from build123d import *

# Parameters (mm, degrees)
F3_DEPTH = 3.15
F4_R     = 0.79999
F5_R     = 0.6


# Not quite as in the source:
# - a fillet or chamfer is up to 0.001 mm smaller than in the source, because OpenCascade refuses the exact size


with BuildPart() as f1:
    # F0 (on Front) → F1 (revolve)
    with BuildSketch(Plane.XZ):
        Polygon((0, 24.5), (0, 0), (4, 0), (4, 15), (2.5, 15), (2.5, 24.5), align=None)
    revolve(axis=Axis((0, 0, -0.3548332296), (0, 0, -1)))

    # F2 (on Front) → F3 (join, symmetric)
    with BuildSketch(Plane.XZ):
        with BuildLine():
            ThreePointArc((-2.9166666667, 29.7373446176), (-1.4719601444, 23.2806810659), (4, 27))
            ThreePointArc((4, 27), (3.7193189341, 28.4719601444), (2.9166666667, 29.7373446176))
            Line((2.9166666667, 29.7373446176), (1.75, 28.6424067706))
            ThreePointArc((1.75, 28.6424067706), (2.2315913604, 27.8831760866), (2.4, 27))
            ThreePointArc((2.4, 27), (-0.8831760866, 24.7684086396), (-1.75, 28.6424067706))
            Line((-1.75, 28.6424067706), (-2.9166666667, 29.7373446176))
        make_face()
    extrude(amount=F3_DEPTH, both=True)

    # F4 (radius 0.8 in the source; OpenCascade refuses exactly that, so slightly less here)
    f4_edges = [f1.edges().sort_by_distance(p)[0] for p in [
        (2.916667, -1.575, 29.737345),
        (2.916667, 1.575, 29.737345),
        (1.75, -1.575, 28.642407),
        (1.75, 1.575, 28.642407),
        (-1.75, 1.575, 28.642407),
        (-1.75, -1.575, 28.642407),
        (-2.916667, -1.575, 29.737345),
        (-2.916667, 1.575, 29.737345),
    ]]
    fillet(f4_edges, radius=F4_R)

    # F5
    f5_edges = [f1.edges().sort_by_distance(p)[0] for p in [
        (-4, 0, 0),
        (-4, 0, 15),
    ]]
    fillet(f5_edges, radius=F5_R)


solid = f1.part
Here's how the part is built. I have some questions about the finished solid (model axes, mm). A direction names the side the tool comes from. Coordinates: 2 decimals unless noted, no trailing zeros. Order: outer loops, then holes, each group sorted by start corner. A loop starts at its lowest first (then second) coordinate and runs counter-clockwise, first axis right, second up. Notation, with made-up numbers: M 2.5,30 L 17.5,30 A17 cw 17.5,48 Z; hole C -21,18.5 d2. An arc over 180 degrees is marked long. Answer as CSV lines item,"result".
Item 1: On a 3-axis mill with a long thin cutter (end or side, diameter ignored), from which of +Z, -Z, +X, -X, +Y, -Y can I reach the whole of each face in a straight line? I mean faces 1 (the face through (0, -3.15, 24)), 2 (the face through (-0.867, 3.905, 7.597)), 3 (the face through (2.016, -0.044, 28.656)), 4 (the face through (0, 3.15, 24)). Say none if no direction works.
Results found:
face 1,"+Z, +X, -X, -Y"
face 2,"-Z"
face 3,"+Y, -Y"
face 4,"+Z, +X, -X, +Y"
Item 2: We'd pull the mould along X, two halves only. Please class faces 5 (the face through (-2.943, 0.044, 29.325)), 6 (the face through (-2, -2, 15)), 7 (the face through (-2.5, -0.1, 19.5)): +X half, -X half, draft (parallel to the pull), parting line (faces both ways), or undercut.
Results found:
face 5,"undercut"
face 6,"draft"
face 7,"parting line"
Item 3: Imagine slicing it at A-A on x = 0. Write out the boundary of the cut face in (y, z), plus the area to 3 significant figures.
Results found:
outline,"M -4,0.6 A0.6 ccw -3.4,0 L 3.4,0 A0.6 ccw 4,0.6 L 4,14.4 A0.6 ccw 3.4,15 L 2.5,15 L 2.5,23 L 3.15,23 L 3.15,24.6 L -3.15,24.6 L -3.15,23 L -2.5,23 L -2.5,15 L -3.4,15 A0.6 ccw -4,14.4 Z"
area,"170 mm2"
Item 4: If I drill on line 1 (X direction, y = 0.5, z = 27); line 2 (Z direction, x = 0, y = -1.5); line 3 (Z direction, x = -3.25, y = -0.5), over which ranges is the centre line in solid material (lowest first)?
Results found:
line 1,"-4 to -2.4, 2.4 to 4"
line 2,"0 to 24.6"
line 3,"0 to 15, 24.67 to 29.2"
Item 5: Imagine slicing it at B-B on z = 25.75. Write out the boundary of the cut face in (x, y).
Results found:
outline,"M -3.8,-3.15 L -2.05,-3.15 L -2.05,3.15 L -3.8,3.15 Z; M 2.05,-3.15 L 3.8,-3.15 L 3.8,3.15 L 2.05,3.15 Z"
Item 6: Imagine slicing it at D-D on z = 2.25. Write out the boundary of the cut face in (x, y).
Results found:
outline,"C 0,0 d8"
Item 7: For pin 1 (1 mm diameter, centred on x = 0.5, y = -1, fed in from +Z); pin 2 (4 mm diameter, centred on x = 1, z = 19, fed in from +Y); pin 3 (3 mm diameter, centred on x = 0, y = 3, fed in from +Z), each with a flat end and sliding along its axis, tell me the tip position at first contact or that it passes through.
Results found:
pin 1,"z = 24.82"
pin 2,"y = 2.5"
pin 3,"z = 25.13"
